For this review, use the dimensioned drawing (mm, ordinates from the lowest corner) and the shaded views. Give positions to 0.01 mm unless a question says otherwise; leave off trailing zeros. Order: outer loops, then holes, each group sorted by start corner. A loop starts at its lowest first (then second) coordinate and runs counter-clockwise, first axis right, second up. Notation, with made-up numbers: (41.5, -27.5) -> (77.5, -27.5) arc R22 cw to (77.5, -17.5) -> close; hole circle Ø5 at (22, -18.75). An arc over 180 degrees is marked (long way). One line per item, written item: value. Start each with the question number.
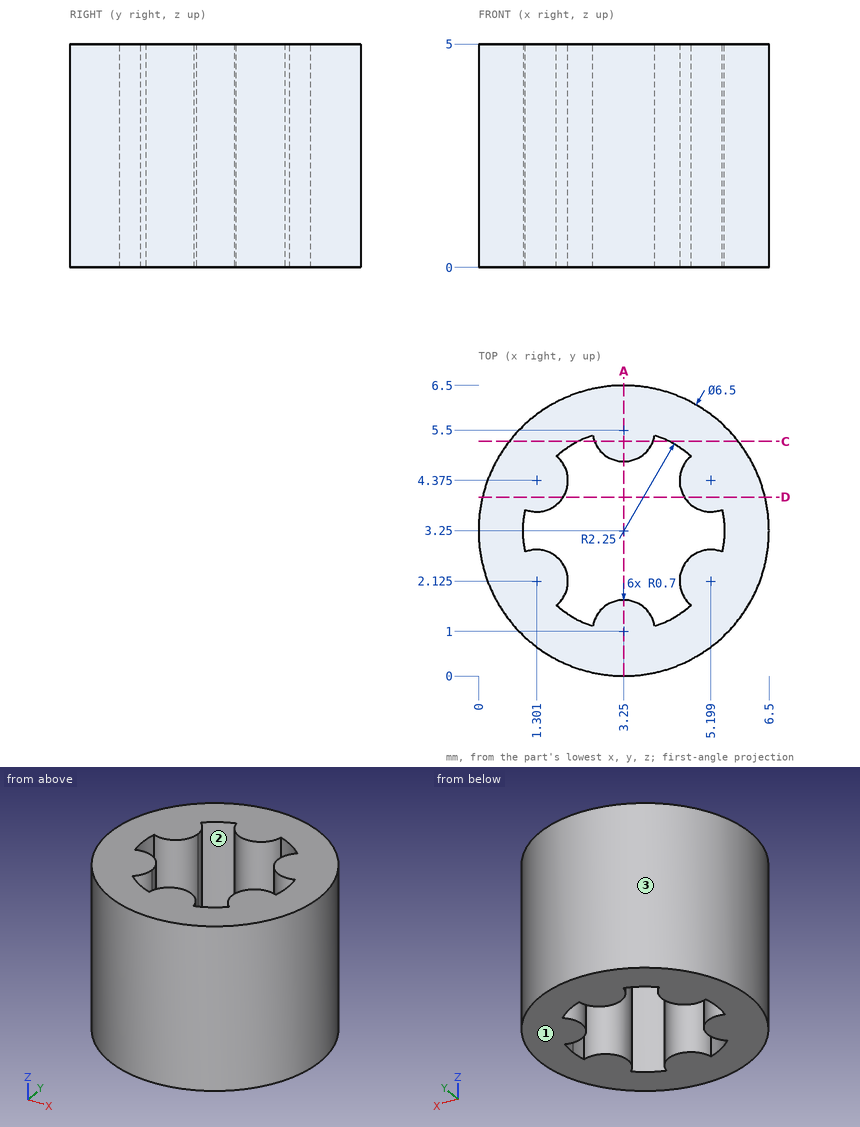
Q1. Take a section at D-D (y = 4). State the section outline as (x, z) points.
Q2. Mouldability with a two-part tool opening along Y and no side actions: class the marked faces 1, 2 and 3 as pulls with the +Y half, pulls with the -Y half, needs draft (parallel to the pull), parting line crosses it, or undercut.
Q3. For line 1 along X through (y, z) = (5, 3.7) (1 decimal); line 2 along Y through (x, z) = (3.25, 2.55); line 3 along X through (y, z) = (4, 4.6), list the stretches that pass through material, from the lowest coordinate up.
Q4. Take a section at A-A (x = 3.25). State the section outline as (y, z) points, and give its area (3 significant figures).
Q5. Take a section at C-C (y = 5.25). State the section outline as (x, z) points.
Q6. For pin 1 Ø2 at (y, z) = (5.5, 3) entering from -X, flat-tipped, find the tip position at first contact; note if it passes through.
Answers below:
1. outline: (0.09, 0) -> (1.89, 0) -> (1.89, 5) -> (0.09, 5) -> close; (4.61, 0) -> (6.41, 0) -> (6.41, 5) -> (4.61, 5) -> close
2. face 1: needs draft
2. face 2: undercut
2. face 3: parting line crosses it
3. line 1: x = 0.5 to 1.8, 2.8 to 3.7, 4.7 to 6
3. line 2: y = 0 to 1.7, 4.8 to 6.5
3. line 3: x = 0.09 to 1.89, 4.61 to 6.41
4. outline: (0, 0) -> (1.7, 0) -> (1.7, 5) -> (0, 5) -> close; (4.8, 0) -> (6.5, 0) -> (6.5, 5) -> (4.8, 5) -> close
4. area: 17.0 mm²
5. outline: (0.69, 0) -> (2.22, 0) -> (2.22, 5) -> (0.69, 5) -> close; (2.6, 0) -> (3.9, 0) -> (3.9, 5) -> (2.6, 5) -> close; (4.28, 0) -> (5.81, 0) -> (5.81, 5) -> (4.28, 5) -> close
6. pin 1: stops at x = 0.25
